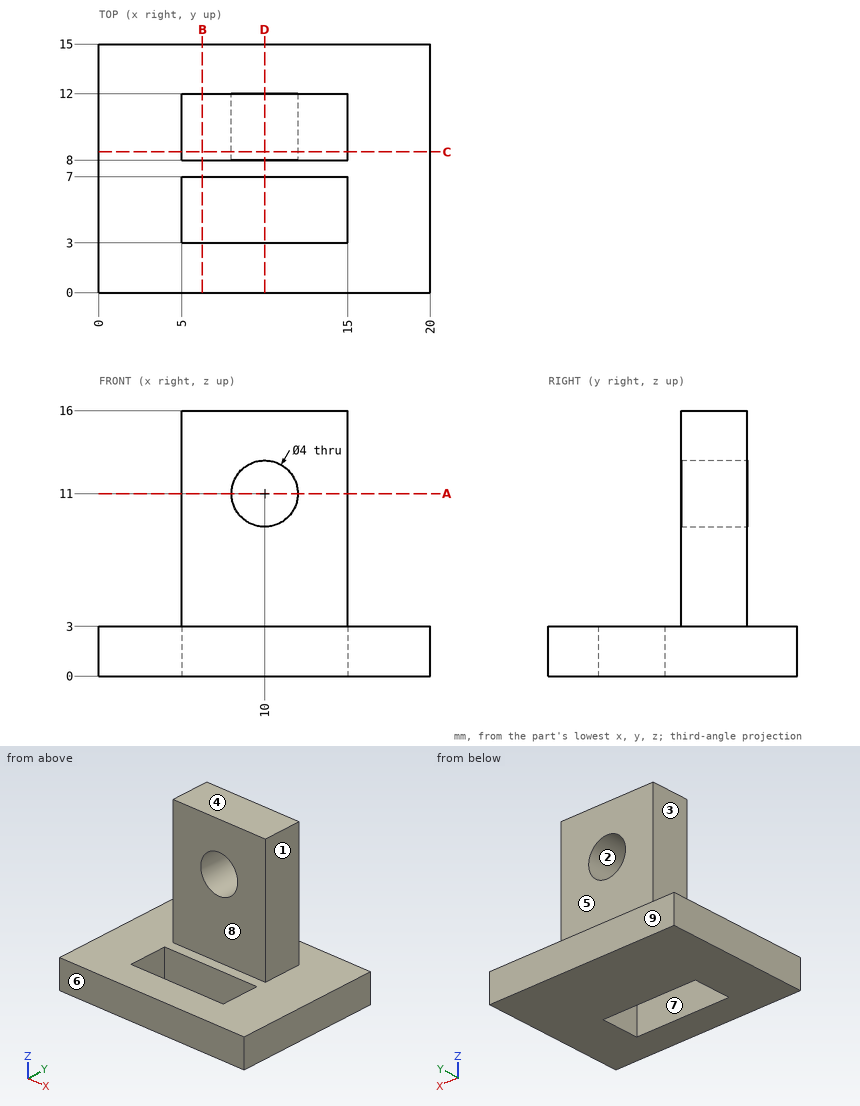
Verification items for this drawing (mm, ordinates from the low corner). A direction names the side the tool comes from. Give positions to 0.01 mm unless a question says otherwise; leave off trailing zeros. Loops run counter-clockwise (first coordinate to the right, second up) from the corner with the lowest first, then second, coordinate; pieces in that order, holes last. Notation, with made-up numbers: M 57,34.5 L 65,34.5 A20 cw 65,58.5 Z; hole C 52.5,16 d4. An arc over 180 degrees is marked long. Write item = value, one per line. Start each with the question number.
1. Go/stop test with flat-tipped pins: P1, Ø3, axis at x = 7, z = 5.5, coming from the -Y side; P2, Ø5, axis at x = 8, z = 9, coming from the +Y side; P3, Ø2, axis at x = 4, y = 3, coming from the +Z side. Record where each tip stops, or that it passes through.
2. Thickness scan on probe 1 along Z at (x, y) = (10, 10.25); probe 2 along Z at (x, y) = (17.5, 9); probe 3 along Y at (x, z) = (7, 11.75). Record the ranges inside material, lowest first.
3. Draft check along X on the marked faces 1, 2, 3 and 4. Enter one of: +X half, -X half, draft (parallel to the pull), parting line (faces both ways), or undercut.
4. Section check C-C, the plane y = 8.5. Enter the section's corners in (x, z), plus the area to 3 significant figures.
5. Tool access check on the marked faces 5, 6, 7, 8 and 9. Record the directions out of +Z, -Z, +X, -X, +Y, -Y that give a thin tool (end or side, any length) a straight path to the whole face; none if there is none.
6. Section check A-A, the plane z = 11. Enter the section's corners in (x, y).
7. Section check B-B, the plane x = 6.25. Enter the section's corners in (y, z).
8. Section check D-D, the plane x = 10. Enter the section's corners in (y, z).
Values follow:
q1.P1 = 8
q1.P2 = 12
q1.P3 = 3
q2.probe_1 = 0 to 9, 13 to 16
q2.probe_2 = 0 to 3
q2.probe_3 = 8 to 12
q3.face_1 = +X half
q3.face_2 = undercut
q3.face_3 = -X half
q3.face_4 = draft
q4.outline = M 0,0 L 20,0 L 20,3 L 15,3 L 15,16 L 5,16 L 5,3 L 0,3 Z; hole C 10,11 d4
q4.area = 177 mm^2
q5.face_5 = +Z, +X, -X, +Y
q5.face_6 = +Z, -Z, +X, -X, -Y
q5.face_7 = +Z, -Z
q5.face_8 = +Z, +X, -X, -Y
q5.face_9 = +Z, -Z, +X, -X, +Y
q6.outline = M 5,8 L 8,8 L 8,12 L 5,12 Z; M 12,8 L 15,8 L 15,12 L 12,12 Z
q7.outline = M 0,0 L 3,0 L 3,3 L 0,3 Z; M 7,0 L 15,0 L 15,3 L 12,3 L 12,16 L 8,16 L 8,3 L 7,3 Z
q8.outline = M 0,0 L 3,0 L 3,3 L 0,3 Z; M 7,0 L 15,0 L 15,3 L 12,3 L 12,9 L 8,9 L 8,3 L 7,3 Z; M 8,13 L 12,13 L 12,16 L 8,16 Z
